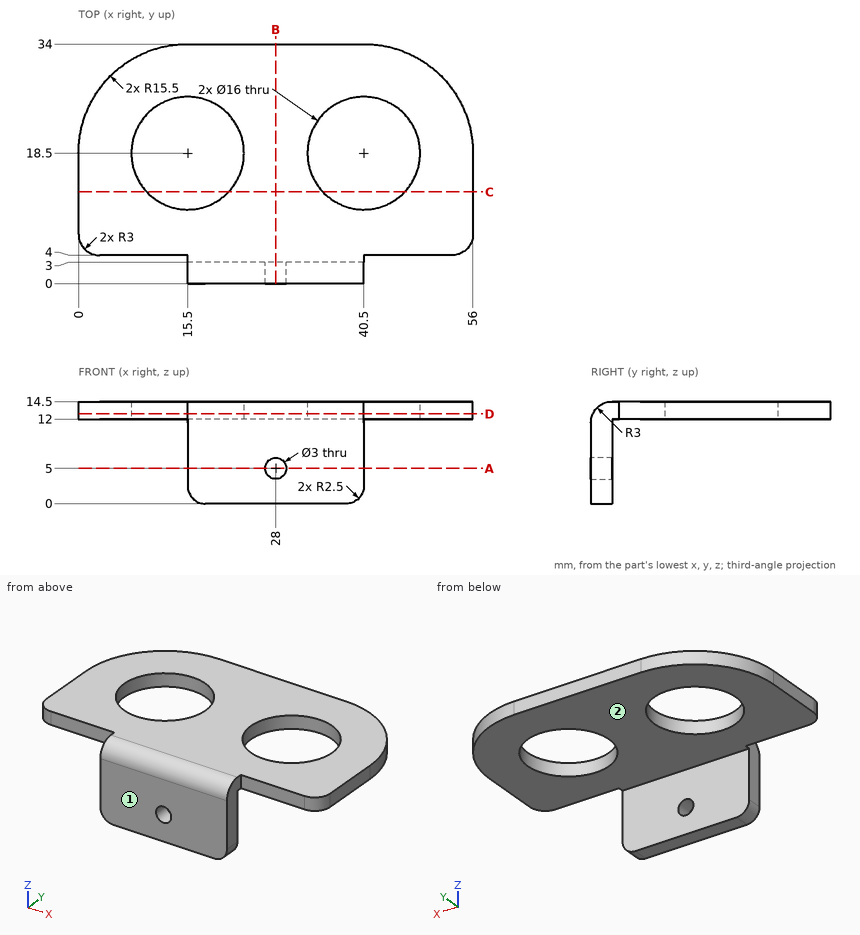
Can you work these out from the drawing? Everything is in mm from the part's minimum corner. A direction names the side the tool comes from. Coordinates: 2 decimals unless noted, no trailing zeros. Write each loop counter-clockwise with the first axis right and the second up, starting at its lowest first coordinate (ties: lowest second). Pieces come first, ordered by that corner, then holes. Notation, with made-up numbers: (86, 8) -> (99, 8) arc R21 cw to (99, 32) -> close; hole circle Ø2 at (42.5, 78.5). An arc over 180 degrees is marked (long way). Write each question's results on one line, items separated by ' | '. Start each with the question number.
Item 1: Please list where these lines run through material, in increasing order: probe 1 along X at (y, z) = (1.15, 5); probe 2 along Z at (x, y) = (21, 8.5); probe 3 along X at (y, z) = (12, 12.25).
Item 2: If we section it at D-D, the plane z = 12.75: Write out the boundary of the cut face in (x, y), and give its area (3 significant figures).
Item 3: On a 3-axis mill with a long thin cutter (end or side, diameter ignored), from which of +Z, -Z, +X, -X, +Y, -Y can I reach the whole of each face in a straight line? I mean the marked faces 1 and 2. Say none if no direction works.
Item 4: If we section it at C-C, the plane y = 13: Write out the boundary of the cut face in (x, z), and give its area (3 significant figures).
Item 5: If we section it at A-A, the plane z = 5: Write out the boundary of the cut face in (x, y).
Item 6: If we section it at B-B, the plane x = 28: Write out the boundary of the cut face in (y, z).
Item 7: I'm going to push flat-ended pins straight in: P1, Ø3.5, axis at x = 28, z = 5, coming from the +Y side; P2, Ø10, axis at x = 20, y = 5, coming from the -Z side; P3, Ø1.2, axis at y = 1.5, z = 10.5, coming from the +X side; P4, Ø18.5, axis at x = 40.5, y = 18.5, coming from the -Z side. Where does each tip first touch, or does it pass through?
Answer block:
1) probe 1: 15.5 to 26.5, 29.5 to 40.5 | probe 2: 12 to 14.5 | probe 3: 0 to 10.84, 20.16 to 35.84, 45.16 to 56
2) outline: (0, 7) arc R3 ccw to (3, 4) -> (15.5, 4) -> (15.5, 0.27) -> (40.5, 0.27) -> (40.5, 4) -> (53, 4) arc R3 ccw to (56, 7) -> (56, 18.5) arc R15.5 ccw to (40.5, 34) -> (15.5, 34) arc R15.5 ccw to (0, 18.5) -> close; hole circle Ø16 at (15.5, 18.5); hole circle Ø16 at (40.5, 18.5) | area: 1,260 mm²
3) face 1: +Z, -Z, +X, -X, -Y | face 2: -Z, +X, -X, +Y
4) outline: (0, 12) -> (9.69, 12) -> (9.69, 14.5) -> (0, 14.5) -> close; (21.31, 12) -> (34.69, 12) -> (34.69, 14.5) -> (21.31, 14.5) -> close; (46.31, 12) -> (56, 12) -> (56, 14.5) -> (46.31, 14.5) -> close | area: 81.9 mm²
5) outline: (15.5, 0) -> (26.5, 0) -> (26.5, 3) -> (15.5, 3) -> close; (29.5, 0) -> (40.5, 0) -> (40.5, 3) -> (29.5, 3) -> close
6) outline: (0, 0) -> (3, 0) -> (3, 3.5) -> (0, 3.5) -> close; (0, 6.5) -> (3, 6.5) -> (3, 12) -> (34, 12) -> (34, 14.5) -> (3, 14.5) arc R3 ccw to (0, 11.5) -> close
7) P1: y = 3 | P2: z = 0 | P3: x = 40.5 | P4: z = 12
